from build123d import *

# Parameters (mm, degrees)
SKETCH_1_W      = 41
SKETCH_1_H      = 15.5
EXTRUDE_1_DEPTH = 1
SKETCH_2_W      = 5.5
SKETCH_2_H      = 11
EXTRUDE_2_DEPTH = 27
SKETCH_3_W      = 5.5
SKETCH_3_H      = 11
EXTRUDE_3_DEPTH = 2
SKETCH_4_W      = 6
SKETCH_4_H      = 6.05
EXTRUDE_4_DEPTH = 9.7
SKETCH_5_R      = 2.64
EXTRUDE_5_DEPTH = 3.4


with BuildPart() as part:
    # 草图1 → 凸台-拉伸1 (new body)
    with BuildSketch(Plane(origin=(0, 0, 0), x_dir=(1, 0, 0), z_dir=(0, 1, 0))):
        Rectangle(SKETCH_1_W, SKETCH_1_H)
    extrude(amount=EXTRUDE_1_DEPTH)

    # 草图2 → 凸台-拉伸2 (add)
    with BuildSketch(Plane(origin=(0, 1, 0), x_dir=(1, 0, 0), z_dir=(0, 1, 0))):
        with Locations((17.75, 0)):
            Rectangle(SKETCH_2_W, SKETCH_2_H)
    extrude(amount=EXTRUDE_2_DEPTH)

    # 草图3 → 凸台-拉伸3 (add)
    with BuildSketch(Plane.XZ):
        with Locations((17.75, 0)):
            Rectangle(SKETCH_3_W, SKETCH_3_H)
    extrude(amount=EXTRUDE_3_DEPTH)

    # 草图4 → 凸台-拉伸4 (add)
    with BuildSketch(Plane.XZ):
        with Locations((-17.5, 0)):
            Rectangle(SKETCH_4_W, SKETCH_4_H)
    extrude(amount=EXTRUDE_4_DEPTH)

    # 草图5 → 凸台-拉伸5 (add)
    with BuildSketch(Plane.ZY.offset(20.5)):
        with Locations(Location((0, -6.679228268, 0), (0, 0, 180))):
            Circle(SKETCH_5_R)
    extrude(amount=EXTRUDE_5_DEPTH)


solid = part.part
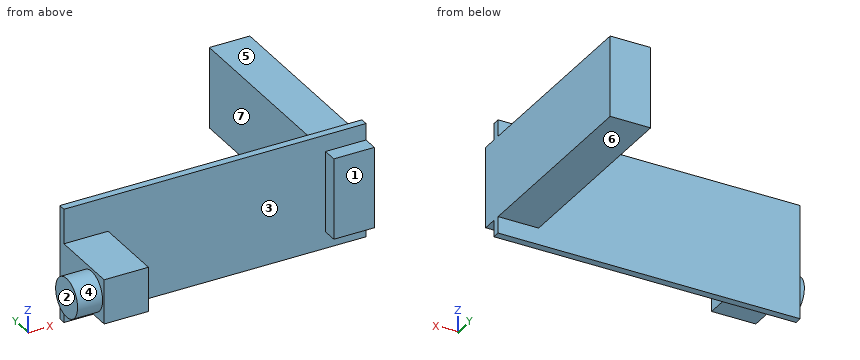
For this review, take the finished solid that the model builds, in its own axes (mm). Face numbers are marked on the shaded views. A direction names the side the tool comes from. Round coordinates to 2 decimals unless told otherwise and drop trailing zeros. Order: outer loops, then holes, each group sorted by start corner. A loop starts at its lowest first (then second) coordinate and runs counter-clockwise, first axis right, second up. Notation, with made-up numbers: M 86,70.25 L 105,70.25 A9 ccw 105,83.25 Z; hole C 53,21.5 d5. An arc over 180 degrees is marked long. Write each question's results on one line, items separated by ' | '. Start each with the question number.
1. Draft analysis for pull direction X (two halves, no side actions). For the marked faces 1, 2 and 3, state which applies: pulls with the +X half, pulls with the -X half, needs draft (parallel to the pull), parting line crosses it, or undercut.
2. To check wall thickness, follow L1, parallel to Y at x = 0.5, z = -1.5; L2, parallel to X at y = 6.5, z = -2.75; L3, parallel to X at y = -6.5, z = -2.25. State the ranges of each line that lie inside material, in increasing order. Write a range as [from, to].
3. Add section B-B (x = 9.5). State the section outline as (y, z) points.
4. Tool access review of the marked faces 4, 5, 6 and 7: name each direction out of +Z, -Z, +X, -X, +Y, -Y from which nothing blocks a thin tool from reaching the whole face with its end or side.
5. Add section C-C (y = 10). State the section outline as (x, z) points.
6. Clearance check with flat-ended pins moving along their axes: pin 1 Ø2 at (y, z) = (-0.5, 0) entering from -X; pin 2 Ø5 at (x, y) = (-19, -4) entering from +Z (3 decimals); pin 3 Ø1.8 at (y, z) = (-4.5, 0) entering from +X. State where each tip first meets the part, or that it passes through.
7. Add section A-A (z = 0). State the section outline as (x, y) points.
Output values:
1) face 1: needs draft | face 2: pulls with the -X half | face 3: undercut
2) L1: [0, 1] | L2: [15, 20.5] | L3: [-23.9, -14.5]
3) outline: M 0,-7.75 L 1,-7.75 L 1,7.75 L 0,7.75 Z
4) face 4: -X | face 5: +Z, +X, -X, +Y | face 6: -Z, +X, -X, +Y | face 7: +Z, -Z, -X, +Y
5) outline: M 15,-5.5 L 20.5,-5.5 L 20.5,5.5 L 15,5.5 Z
6) pin 1: x = -20.5 | pin 2: z = 3.025 | pin 3: x = -14.5
7) outline: M -23.9,-9.32 L -20.5,-9.32 L -20.5,-9.7 L -14.5,-9.7 L -14.5,0 L 15,0 L 15,-2 L 20.5,-2 L 20.5,28 L 15,28 L 15,1 L -20.5,1 L -20.5,-4.04 L -23.9,-4.04 Z
